Verification items for the finished model (mm, model axes). A direction names the side the tool comes from. Round coordinates to 2 decimals unless told otherwise and drop trailing zeros. Loops run counter-clockwise (first coordinate to the right, second up) from the corner with the lowest first, then second, coordinate; pieces in that order, holes last. Notation, with made-up numbers: (-34.75, -9.75) -> (-29.75, -9.75) arc R21 ccw to (-29.75, 27.25) -> close; hole circle Ø6 at (77, 8). An arc over 180 degrees is marked (long way). Use CSV: the item, a comma, the result in double quotes. Start each with the question number.
```python
from build123d import *

# Parameters (mm, degrees)
F0_R     = 1.85
F0_R_2   = 1.35
F1_DEPTH = 6.5
F2_START = 3.35
F2_DEPTH = 3.15
F3_R     = 2
F4_R     = 2


with BuildPart() as f1:
    # F0 (on Top) → F1 (new body)
    with BuildSketch(Plane.XY):
        with BuildLine():
            Line((-7.4, -10.4), (-12.4, -10.4))
            Line((-12.4, -10.4), (-12.4, -23.65))
            Line((-12.4, -23.65), (-1.303840481, -23.65))
            ThreePointArc((-1.303840481, -23.65), (-0.1765153684, -21.9615896277), (1.35, -23.3))
            ThreePointArc((1.35, -23.3), (1.3384103723, -23.4765153684), (1.303840481, -23.65))
            Line((1.303840481, -23.65), (12.4, -23.65))
            Line((12.4, -23.65), (12.4, -10.4))
            Line((12.4, -10.4), (7.4, -10.4))
            Line((7.4, -10.4), (7.4, -20.25))
            Line((7.4, -20.25), (7.4, -21.45))
            Line((7.4, -21.45), (-7.4, -21.45))
            Line((-7.4, -21.45), (-7.4, -20.25))
            Line((-7.4, -20.25), (-7.4, -10.4))
        make_face()
        Polygon((-24.4, -5.2615826042), (-24.4, -10.4), (-12.4, -10.4), (-7.4, -10.4), (-7.4, 7.05), (-4, 7.05), (-4, 7.85), (4, 7.85), (4, 7.05), (7.4, 7.05), (7.4, -10.4), (12.4, -10.4), (24.4, -10.4), (24.4, 10.4), (9.4, 10.4), (9.4, 13.65), (-9.4, 13.65), (-9.4, 10.4), (-24.4, 10.4), align=None)
        with Locations((-19.4, -5.4)):
            Circle(F0_R, mode=Mode.SUBTRACT)
        with Locations((-19.4, 5.4)):
            Circle(F0_R, mode=Mode.SUBTRACT)
        with Locations((19.4, 0)):
            Circle(F0_R, mode=Mode.SUBTRACT)
        with Locations((0, 9.8)):
            Circle(F0_R_2, mode=Mode.SUBTRACT)
    extrude(amount=F1_DEPTH)

    # F0 (on Top) → F2 (join)
    with BuildSketch(Plane.XY.offset(F2_START)):
        with BuildLine():
            Line((-1.303840481, -23.65), (-12.4, -23.65))
            Line((-12.4, -23.65), (-12.4, -27.15))
            Line((-12.4, -27.15), (12.4, -27.15))
            Line((12.4, -27.15), (12.4, -23.65))
            Line((12.4, -23.65), (1.303840481, -23.65))
            ThreePointArc((1.303840481, -23.65), (0, -24.65), (-1.303840481, -23.65))
        make_face()
    extrude(amount=F2_DEPTH)

    # F3
    f3_edges = [f1.edges().sort_by_distance(p)[0] for p in [
        (-24.4, -10.4, 3.25),
        (-24.4, 10.4, 3.25),
        (24.4, -10.4, 3.25),
        (24.4, 10.4, 3.25),
        (9.4, 13.65, 3.25),
        (-12.4, -27.15, 4.925),
        (-12.4, -23.65, 1.675),
        (12.4, -27.15, 4.925),
        (12.4, -23.65, 1.675),
        (12.4, -10.4, 3.25),
        (-12.4, -10.4, 3.25),
        (-9.4, 13.65, 3.25),
    ]]
    fillet(f3_edges, radius=F3_R)

    # F4
    f4_edges = [f1.edges().sort_by_distance(p)[0] for p in [
        (-9.4, 10.4, 3.25),
        (9.4, 10.4, 3.25),
    ]]
    fillet(f4_edges, radius=F4_R)


solid = f1.part
```
Q1. Release check for a two-part mould opening along Y. For faces 6 (the face through (-17.69, 4.69, 3.2)), 7 (the face through (8.66, 13.203, 3.296)), 8 (the face through (24.4, 0, 3)), 9 (the face through (0, 7.85, 3)) record: +Y half, -Y half, draft (parallel to the pull), parting line (faces both ways), or undercut.
Q2. Cross-section at A-A (x = 5). Record the boundary of the cut face in (y, z), and give its area (3 significant figures).
Q3. Thickness scan on L1, parallel to Y at x = -19.4, z = 4.5; L2, parallel to X at y = -15, z = 5.25; L3, parallel to X at y = 6.5, z = 3.25. Record the ranges inside material, lowest first. Write a range as from..to.
Q4. Depth check by flat-ended pin: pin 1 Ø2 at (y, z) = (-17, 3.5) entering from -X; pin 2 Ø2.5 at (x, z) = (-5.5, 2) entering from -Y; pin 3 Ø2 at (x, z) = (-19.5, 5) entering from -Y. Enter the tip coordinate at first touch or a pass-through.
Q5. Cross-section at C-C (x = -19.4). Record the boundary of the cut face in (y, z).
Q6. Tool access check on faces 1 (the face through (-17, 10.4, 3)), 2 (the face through (17, 10.4, 3)), 3 (the face through (7.4, -7, 3)), 4 (the face through (18, -10.4, 3)), 5 (the face through (-12.4, -19, 3)). Record the directions out of +Z, -Z, +X, -X, +Y, -Y that give a thin tool (end or side, any length) a straight path to the whole face; none if there is none.
Q7. Cross-section at B-B (y = -5.4). Record the boundary of the cut face in (x, z).
Q8. Cross-section at D-D (y = -13). Record the boundary of the cut face in (x, z), and give its area (3 significant figures).
Answer list:
1,face 6,"undercut"
1,face 7,"+Y half"
1,face 8,"draft"
1,face 9,"undercut"
2,outline,"(-27.15, 3.35) -> (-23.65, 3.35) -> (-23.65, 0) -> (-21.45, 0) -> (-21.45, 6.5) -> (-27.15, 6.5) -> close; (7.05, 0) -> (13.65, 0) -> (13.65, 6.5) -> (7.05, 6.5) -> close"
2,area,"68.2 mm2"
3,L1,"y = -10.4..-7.25, -3.55..3.55, 7.25..10.4"
3,L2,"x = -12.4..-7.4, 7.4..12.4"
3,L3,"x = -24.4..-20.89, -17.91..-7.4, 7.4..24.4"
4,pin 1,"stops at x = -12.4"
4,pin 2,"stops at y = -23.65"
4,pin 3,"stops at y = -10.4"
5,outline,"(-10.4, 0) -> (-7.25, 0) -> (-7.25, 6.5) -> (-10.4, 6.5) -> close; (-3.55, 0) -> (3.55, 0) -> (3.55, 6.5) -> (-3.55, 6.5) -> close; (7.25, 0) -> (10.4, 0) -> (10.4, 6.5) -> (7.25, 6.5) -> close"
6,face 1,"+Z, -Z, -X, +Y"
6,face 2,"+Z, -Z, +X, +Y"
6,face 3,"+Z, -Z"
6,face 4,"+Z, -Z, +X, -Y"
6,face 5,"+Z, -Z, -X, -Y"
7,outline,"(-24.4, 0) -> (-21.25, 0) -> (-21.25, 6.5) -> (-24.4, 6.5) -> close; (-17.55, 0) -> (-7.4, 0) -> (-7.4, 6.5) -> (-17.55, 6.5) -> close; (7.4, 0) -> (24.4, 0) -> (24.4, 6.5) -> (7.4, 6.5) -> close"
8,outline,"(-12.4, 0) -> (-7.4, 0) -> (-7.4, 6.5) -> (-12.4, 6.5) -> close; (7.4, 0) -> (12.4, 0) -> (12.4, 6.5) -> (7.4, 6.5) -> close"
8,area,"65.0 mm2"
